from build123d import *

# Parameters (mm, degrees)
SKETCH2_R       = 2.5
SKETCH2_R_2     = 1
MAIN_BODY_DEPTH = 5
FILLET1_R       = 3
SKETCH2_3_R     = 2.5
SKETCH2_3_R_2   = 1.375
STRAWS_DEPTH    = 10


with BuildPart() as part:
    # Sketch2 → Main Body (new body)
    with BuildSketch(Plane.XY):
        Polygon((141.081115161, -34.767752), (134.096872, -34.767752), (134.096872, -114.226250672), (152.171772965, -114.226250672), (152.171772965, -100.344538887), (141.081115161, -100.344538887), align=None)
        with Locations((137.596872, -96.267752)):
            Circle(SKETCH2_R, mode=Mode.SUBTRACT)
        with Locations((136.368346882, -91.088967224)):
            Circle(SKETCH2_R_2, mode=Mode.SUBTRACT)
        with Locations((136.368346882, -88.548967224)):
            Circle(SKETCH2_R_2, mode=Mode.SUBTRACT)
        with Locations((136.368346882, -86.008967224)):
            Circle(SKETCH2_R_2, mode=Mode.SUBTRACT)
        with Locations((136.368346882, -83.468967224)):
            Circle(SKETCH2_R_2, mode=Mode.SUBTRACT)
        with Locations((136.368346882, -80.928967224)):
            Circle(SKETCH2_R_2, mode=Mode.SUBTRACT)
        with Locations((136.368346882, -78.388967224)):
            Circle(SKETCH2_R_2, mode=Mode.SUBTRACT)
        with Locations((136.368346882, -75.848967224)):
            Circle(SKETCH2_R_2, mode=Mode.SUBTRACT)
        with Locations((138.883114052, -91.04875221)):
            Circle(SKETCH2_R_2, mode=Mode.SUBTRACT)
        with Locations((138.883114052, -88.50875221)):
            Circle(SKETCH2_R_2, mode=Mode.SUBTRACT)
        with Locations((138.883114052, -85.96875221)):
            Circle(SKETCH2_R_2, mode=Mode.SUBTRACT)
        with Locations((138.883114052, -83.42875221)):
            Circle(SKETCH2_R_2, mode=Mode.SUBTRACT)
        with Locations((138.883114052, -80.88875221)):
            Circle(SKETCH2_R_2, mode=Mode.SUBTRACT)
        with Locations((138.883114052, -78.34875221)):
            Circle(SKETCH2_R_2, mode=Mode.SUBTRACT)
        with Locations((138.883114052, -75.80875221)):
            Circle(SKETCH2_R_2, mode=Mode.SUBTRACT)
        with Locations((136.368346882, -73.308967224)):
            Circle(SKETCH2_R_2, mode=Mode.SUBTRACT)
        with Locations((136.368346882, -70.768967224)):
            Circle(SKETCH2_R_2, mode=Mode.SUBTRACT)
        with Locations((136.368346882, -68.228967224)):
            Circle(SKETCH2_R_2, mode=Mode.SUBTRACT)
        with Locations((136.368346882, -65.688967224)):
            Circle(SKETCH2_R_2, mode=Mode.SUBTRACT)
        with Locations((136.368346882, -63.148967224)):
            Circle(SKETCH2_R_2, mode=Mode.SUBTRACT)
        with Locations((136.368346882, -60.608967224)):
            Circle(SKETCH2_R_2, mode=Mode.SUBTRACT)
        with Locations((136.368346882, -58.068967224)):
            Circle(SKETCH2_R_2, mode=Mode.SUBTRACT)
        with Locations((136.368346882, -55.528967224)):
            Circle(SKETCH2_R_2, mode=Mode.SUBTRACT)
        with Locations((138.883114052, -73.26875221)):
            Circle(SKETCH2_R_2, mode=Mode.SUBTRACT)
        with Locations((138.883114052, -70.72875221)):
            Circle(SKETCH2_R_2, mode=Mode.SUBTRACT)
        with Locations((138.883114052, -68.18875221)):
            Circle(SKETCH2_R_2, mode=Mode.SUBTRACT)
        with Locations((138.883114052, -65.64875221)):
            Circle(SKETCH2_R_2, mode=Mode.SUBTRACT)
        with Locations((138.883114052, -63.10875221)):
            Circle(SKETCH2_R_2, mode=Mode.SUBTRACT)
        with Locations((138.883114052, -60.56875221)):
            Circle(SKETCH2_R_2, mode=Mode.SUBTRACT)
        with Locations((138.883114052, -58.02875221)):
            Circle(SKETCH2_R_2, mode=Mode.SUBTRACT)
        with Locations((138.883114052, -55.48875221)):
            Circle(SKETCH2_R_2, mode=Mode.SUBTRACT)
        with Locations((136.368346882, -52.988967224)):
            Circle(SKETCH2_R_2, mode=Mode.SUBTRACT)
        with Locations((136.368346882, -50.448967224)):
            Circle(SKETCH2_R_2, mode=Mode.SUBTRACT)
        with Locations((136.368346882, -47.908967224)):
            Circle(SKETCH2_R_2, mode=Mode.SUBTRACT)
        with Locations((136.368346882, -45.368967224)):
            Circle(SKETCH2_R_2, mode=Mode.SUBTRACT)
        with Locations((136.368346882, -42.828967224)):
            Circle(SKETCH2_R_2, mode=Mode.SUBTRACT)
        with Locations((137.596872, -38.267752)):
            Circle(SKETCH2_R, mode=Mode.SUBTRACT)
        with Locations((138.883114052, -52.94875221)):
            Circle(SKETCH2_R_2, mode=Mode.SUBTRACT)
        with Locations((138.883114052, -50.40875221)):
            Circle(SKETCH2_R_2, mode=Mode.SUBTRACT)
        with Locations((138.883114052, -47.86875221)):
            Circle(SKETCH2_R_2, mode=Mode.SUBTRACT)
        with Locations((138.883114052, -45.32875221)):
            Circle(SKETCH2_R_2, mode=Mode.SUBTRACT)
        with Locations((138.883114052, -42.78875221)):
            Circle(SKETCH2_R_2, mode=Mode.SUBTRACT)
        with Locations((145.030003125, -104.034694376)):
            Circle(SKETCH2_R_2, mode=Mode.SUBTRACT)
        with BuildLine():
            Line((138.496220073, -105.367628272), (147.819131421, -105.367628272))
            ThreePointArc((147.819131421, -105.367628272), (151.349843906, -104.796920677), (149.692119851, -107.966082833))
            Line((149.692119851, -107.966082833), (149.692119851, -109.599156243))
            ThreePointArc((149.692119851, -109.599156243), (150.237287523, -113.523420313), (148.643073288, -109.896364034))
            Line((148.643073288, -109.896364034), (137.950744717, -109.896364034))
            ThreePointArc((137.950744717, -109.896364034), (136.043263655, -113.333173494), (136.567489161, -109.437620787))
            Line((136.567489161, -109.437620787), (136.567489161, -107.874618377))
            ThreePointArc((136.567489161, -107.874618377), (134.985954912, -104.66245765), (138.496220073, -105.367628272))
        make_face(mode=Mode.SUBTRACT)
        with Locations((139.950003125, -111.497761483)):
            Circle(SKETCH2_R_2, mode=Mode.SUBTRACT)
        with Locations((142.490003125, -111.497761483)):
            Circle(SKETCH2_R_2, mode=Mode.SUBTRACT)
        with Locations((139.950003125, -104.034694376)):
            Circle(SKETCH2_R_2, mode=Mode.SUBTRACT)
        with Locations((142.490003125, -104.034694376)):
            Circle(SKETCH2_R_2, mode=Mode.SUBTRACT)
        with Locations((145.030003125, -111.497761483)):
            Circle(SKETCH2_R_2, mode=Mode.SUBTRACT)
    extrude(amount=MAIN_BODY_DEPTH)

    # Fillet1
    fillet1_edges = [part.edges().sort_by_distance(p)[0] for p in [
        (134.096872, -34.767752, 2.5),
        (141.081115161, -34.767752, 2.5),
        (141.081115161, -100.344538887, 2.5),
        (152.171772965, -100.344538887, 2.5),
        (152.171772965, -114.226250672, 2.5),
        (134.096872, -114.226250672, 2.5),
    ]]
    fillet(fillet1_edges, radius=FILLET1_R)

    # Sketch2<3> → Straws (add)
    # profile 1 of 2: a face of its own
    with BuildSketch(Plane.XY):
        with Locations((137.596872, -38.267752)):
            Circle(SKETCH2_3_R)
        with Locations((137.596872, -38.267752)):
            Circle(SKETCH2_3_R_2, mode=Mode.SUBTRACT)
    # profile 2 of 2: a face of its own
    with BuildSketch(Plane.XY):
        with Locations((137.596872, -96.267752)):
            Circle(SKETCH2_3_R)
        with Locations((137.596872, -96.267752)):
            Circle(SKETCH2_3_R_2, mode=Mode.SUBTRACT)
    extrude(amount=STRAWS_DEPTH)


solid = part.part
Input: part model. Units: mm. Frame: model coordinates. Coordinates: 2 decimals unless noted, no trailing zeros. Loops run counter-clockwise (first coordinate to the right, second up) from the corner with the lowest first, then second, coordinate; pieces in that order, holes last. Notation, with made-up numbers: (-32.75, 88) -> (-11.75, 88) arc R21 ccw to (-11.75, 106) -> close; hole circle Ø7 at (-19, 88.25). An arc over 180 degrees is marked (long way). Write item = value, one per line. Start each with the question number.
Item 1: Cut plane C-C, the plane y = -102. Return loops of the section in (x, z), plus the area to 3 significant figures.
Item 2: First-contact query: P1, Ø2.5, axis at y = -66.5, z = 3.5, coming from the +X side; P2, Ø1.5, axis at y = -44, z = 6.5, coming from the -X side; P3, Ø4, axis at x = 147, z = 5.5, coming from the +Y side; P4, Ø2.5, axis at x = 138.88, y = -60.57, coming from the +Z side. Flat tips, straight axial feed; report the tip coordinate or a pass-through.
Item 3: Mould query, pull axis X, two halves, no side actions, for faces 1 (the face through (138.09, -66.26, 2.46)), 2 (the face through (152.172, -107, 2)). Classes: pulls with the +X half, pulls with the -X half, needs draft (parallel to the pull), parting line crosses it, or undercut.
Item 4: Material intervals for line 1 (Y direction, x = 138, z = 5.25); line 2 (Y direction, x = 145, z = 2.5); line 3 (Z direction, x = 138.75, y = -103.5), sorted ascending.
Item 5: Cut plane A-A, the plane x = 145. Return loops of the section in (y, z).
Item 6: Cut plane B-B, the plane z = 5.75. Return loops of the section in (x, y) (3 decimals), plus the area to 3 significant figures.
Ans:
q1.outline = (134.1, 0) -> (151.85, 0) -> (151.85, 5) -> (134.1, 5) -> close
q1.area = 88.8 mm²
q2.P1 = 141.08
q2.P2 = through
q2.P3 = -100.34
q2.P4 = 5
q3.face_1 = undercut
q3.face_2 = pulls with the +X half
q4.line_1 = -98.74 to -97.58, -94.95 to -93.8, -40.74 to -39.58, -36.95 to -35.8
q4.line_2 = -114.23 to -112.5, -110.5 to -109.9, -105.37 to -105.03, -103.04 to -100.34
q4.line_3 = 0 to 5
q5.outline = (-114.23, 0) -> (-112.5, 0) -> (-112.5, 5) -> (-114.23, 5) -> close; (-110.5, 0) -> (-109.9, 0) -> (-109.9, 5) -> (-110.5, 5) -> close; (-105.37, 0) -> (-105.03, 0) -> (-105.03, 5) -> (-105.37, 5) -> close; (-103.04, 0) -> (-100.34, 0) -> (-100.34, 5) -> (-103.04, 5) -> close
q6.outline = circle Ø5 at (137.597, -96.268); circle Ø5 at (137.597, -38.268); hole circle Ø2.75 at (137.597, -96.268); hole circle Ø2.75 at (137.597, -38.268)
q6.area = 27.4 mm²
